Geometry check sheet. Reference: drawing and pictorial views, mm from the part's lowest x, y, z. Give positions to 0.01 mm unless a question says otherwise; leave off trailing zeros. Write each loop counter-clockwise with the first axis right and the second up, starting at its lowest first coordinate (ties: lowest second). Pieces come first, ordered by that corner, then holes. Notation, with made-up numbers: (34, 57) -> (93, 57) arc R9 cw to (93, 71) -> close; hole circle Ø2 at (6.25, 23.25). An arc over 180 degrees is marked (long way). Return JSON: item names as keys, results as strings.
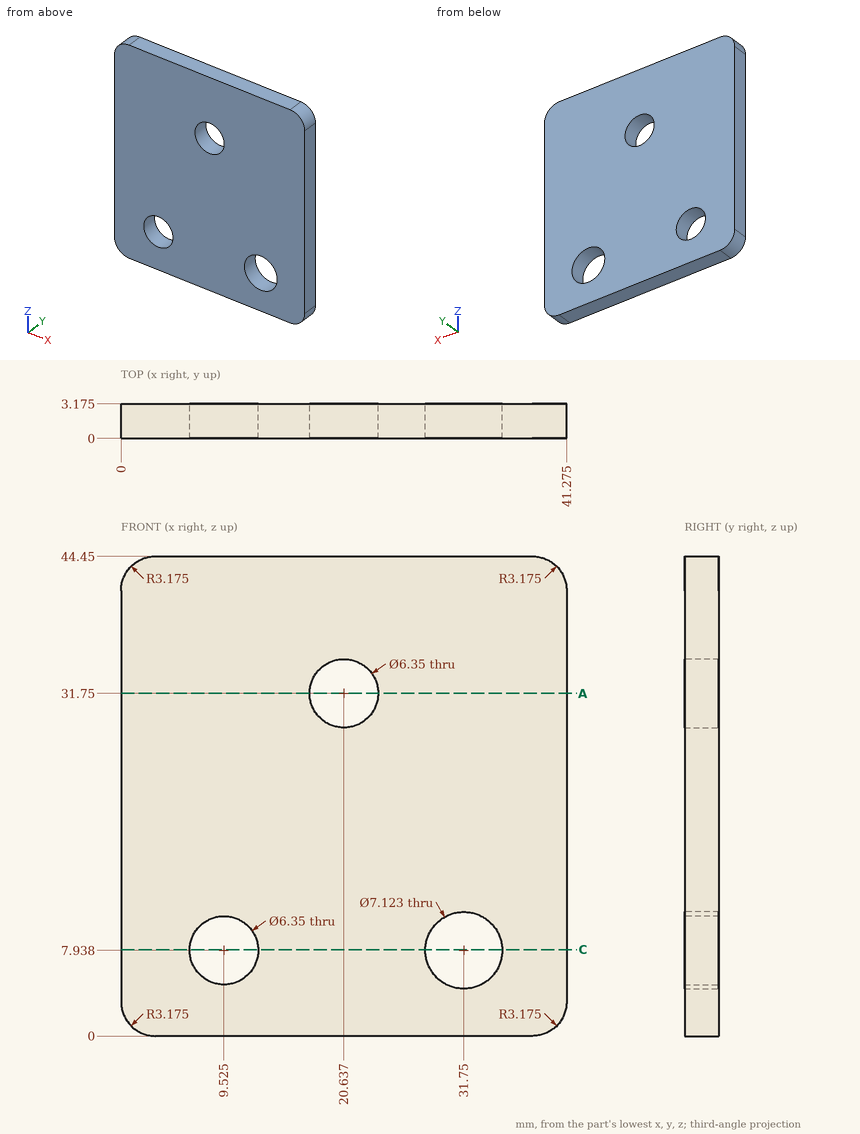
(1) Thickness scan on L1, parallel to X at y = 2.1, z = 31.75 (1 decimal); L2, parallel to Z at x = 19, y = 1.45; L3, parallel to Z at x = 22, y = 1.6. Record the ranges inside material, lowest first.
Reply:
{"L1": "0 to 17.5, 23.8 to 41.3", "L2": "0 to 29.03, 34.47 to 44.45", "L3": "0 to 28.88, 34.62 to 44.45"}
(2) Depth check by flat-ended pin: pin 1 Ø8 at (x, z) = (31.75, 7.94) entering from -Y. Enter the tip coordinate at first touch or a pass-through.
Reply:
{"pin 1": "y = 0"}
(3) Cross-section at A-A on z = 31.75. Enter the section's corners in (x, y) (1 decimal), then the cut area to 3 significant figures.
Reply:
{"outline": "(0, 0) -> (17.5, 0) -> (17.5, 3.2) -> (0, 3.2) -> close; (23.8, 0) -> (41.3, 0) -> (41.3, 3.2) -> (23.8, 3.2) -> close", "area": "111 mm^2"}
(4) Cross-section at C-C on z = 8. State how many separate pieces and enclosed holes the cut face has.
Reply:
{"separate pieces": "3", "enclosed holes": "0"}
